from build123d import *

# Parameters (mm, degrees)
F2_SIZE       = 1.5
F3_W          = 6.717514
F3_H          = 6.717514
F4_DEPTH      = 9
F4_DEPTH_BACK = 3
F5_SIZE       = 0.5


with BuildPart() as f1:
    # F0 (on Front) → F1 (revolve)
    with BuildSketch(Plane.XZ):
        Polygon((0, 80), (0, -80), (4.75, -80), (4.75, -76), (10, -70.75), (10, 68.75), (4.75, 74), (4.75, 80), align=None)
    revolve(axis=Axis((0, 0, 0), (0, 0, -1)))

    # F2
    f2_edges = [f1.edges().sort_by_distance(p)[0] for p in [
        (-4.75, 0, 80),
    ]]
    chamfer(f2_edges, length=F2_SIZE)

    # F3 (on face) → F4 (join, two sides)
    with BuildSketch(Plane.XY.offset(80)) as f4_sk:
        Rectangle(F3_W, F3_H)
    extrude(amount=F4_DEPTH)
    extrude(f4_sk.sketch, amount=-F4_DEPTH_BACK)

    # F5
    f5_edges = [f1.edges().sort_by_distance(p)[0] for p in [
        (-4.75, 0, -80),
    ]]
    chamfer(f5_edges, length=F5_SIZE)


solid = f1.part
Source: CAD feature listing. Evaluate the final solid. Frame: model axes, mm. A direction names the side the tool comes from. Round coordinates to 2 decimals unless told otherwise and drop trailing zeros. Loops run counter-clockwise (first coordinate to the right, second up) from the corner with the lowest first, then second, coordinate; pieces in that order, holes last. Notation, with made-up numbers: M 87,-16.5 L 99,-16.5 A18 ccw 99,-4.5 Z; hole C 26,74.25 d10. An arc over 180 degrees is marked long. Return JSON: item names as keys, results as strings. Group by question number.
1. Material intervals for line 1 along X through (y, z) = (-0.5, -32); line 2 along Y through (x, z) = (-2.75, 79); line 3 along Y through (x, z) = (2.5, 2), sorted ascending. Write a range as from..to.
2. Section query D-D on z = 36. Output: boundary loops of the cut face in (x, y), and give its area (3 significant figures).
3. Mould query, pull axis Z, two halves, no side actions, for faces 4 (the face through (-1.1, 4.96, -75.67)), 5 (the face through (3.359, 0, 84)), 6 (the face through (4.77, -1.5, 73.75)). Classes: released by +Z, released by -Z, zero draft, split by the parting line, or undercut.
4. Pin query (flat end, axial travel): pin 1 (4 mm diameter, centred on y = 6.5, z = -10.5, fed in from +X); pin 2 (2 mm diameter, centred on x = 0, z = 82.5, fed in from -Y); pin 3 (3 mm diameter, centred on x = 5, z = -41, fed in from -Y). Return the tip coordinate at first contact, or that it passes through.
5. Section query A-A on x = 0. Output: boundary loops of the cut face in (y, z), and give its area (3 significant figures).
6. Section query C-C on z = 72.5. Output: boundary loops of the cut face in (x, y), and give its area (3 significant figures).
7. Reachability of faces 1 (the face through (-2.17, 9.76, -0.02)), 2 (the face through (2.192, 4.214, -77.726)), 3 (the face through (2.192, 4.214, 76.282)) from +Z, -Z, +X, -X, +Y, -Y: full face, straight path, thin tool, end or side. Return the list, or none.
Checks:
{
 "1": {"line 1": "x = -9.99..9.99", "line 2": "y = -3.36..3.36", "line 3": "y = -9.68..9.68"},
 "2": {"outline": "C 0,0 d20", "area": "314 mm²"},
 "3": {"face 4": "released by -Z", "face 5": "zero draft", "face 6": "released by +Z"},
 "4": {"pin 1": "stops at x = 8.93", "pin 2": "stops at y = -3.36", "pin 3": "stops at y = -9.37"},
 "5": {"outline": "M -10,-70.75 L -4.75,-76 L -4.75,-79.5 L -4.25,-80 L 4.25,-80 L 4.75,-79.5 L 4.75,-76 L 10,-70.75 L 10,68.75 L 4.75,74 L 4.75,78.5 L 3.36,79.89 L 3.36,89 L -3.36,89 L -3.36,79.89 L -4.75,78.5 L -4.75,74 L -10,68.75 Z", "area": "3,100 mm²"},
 "6": {"outline": "C 0,0 d12.5", "area": "123 mm²"},
 "7": {"face 1": "+Z, -Z", "face 2": "-Z", "face 3": "+Z"}
}
